from build123d import *

# Parameters (mm, degrees)
SKETCH_1_R      = 11.5
SKETCH_1_R_2    = 1.6
SKETCH_1_R_3    = 4.3
SKETCH_1_R_4    = 2.5
EXTRUDE_3_DEPTH = 4
SKETCH_4_W      = 42
SKETCH_4_H      = 2.6
EXTRUDE_4_DEPTH = 6
SKETCH_4_3_W    = 42
SKETCH_4_3_H    = 2.6
EXTRUDE_5_DEPTH = 5
CHAMFER_3_SIZE  = 4
CHAMFER_3_SIZE2 = 22
CHAMFER_4_SIZE  = 22
CHAMFER_4_SIZE2 = 4


with BuildPart() as part:
    # Sketch 1 → Extrude 3 (new body)
    with BuildSketch(Plane.XY):
        with BuildLine():
            Line((-21, 24), (35, 24))
            ThreePointArc((35, 24), (39.242640687, 22.242640687), (41, 18))
            Line((41, 18), (41, -18))
            ThreePointArc((41, -18), (39.242640687, -22.242640687), (35, -24))
            Line((35, -24), (-21, -24))
            Line((-21, -24), (-21, -9.797958971))
            ThreePointArc((-21, -9.797958971), (-21.445079401, -7.530172133), (-22.714285714, -5.598833698))
            ThreePointArc((-22.714285714, -5.598833698), (-25, 0), (-22.714285714, 5.598833698))
            ThreePointArc((-22.714285714, 5.598833698), (-21.445079401, 7.530172133), (-21, 9.797958971))
            Line((-21, 9.797958971), (-21, 24))
        make_face()
        Circle(SKETCH_1_R, mode=Mode.SUBTRACT)
        with Locations((15.5, 15.5)):
            Circle(SKETCH_1_R_2, mode=Mode.SUBTRACT)
        with Locations((15.5, -15.5)):
            Circle(SKETCH_1_R_2, mode=Mode.SUBTRACT)
        with Locations((-15.5, -15.5)):
            Circle(SKETCH_1_R_2, mode=Mode.SUBTRACT)
        with Locations((-15.5, 15.5)):
            Circle(SKETCH_1_R_2, mode=Mode.SUBTRACT)
        with Locations((-17, 0)):
            Circle(SKETCH_1_R_3, mode=Mode.SUBTRACT)
        with Locations((31, 15.5)):
            Circle(SKETCH_1_R_4, mode=Mode.SUBTRACT)
        with Locations(Location((31, -15.5, 0), (0, 0, 180))):
            Circle(SKETCH_1_R_4, mode=Mode.SUBTRACT)
    extrude(amount=EXTRUDE_3_DEPTH)

    # Sketch 4 → Extrude 4 (add)
    with BuildSketch(Plane.XY.offset(4)):
        with Locations((0, 22.7)):
            Rectangle(SKETCH_4_W, SKETCH_4_H)
        with Locations((0, -22.7)):
            Rectangle(SKETCH_4_W, SKETCH_4_H)
    extrude(amount=EXTRUDE_4_DEPTH)

    # Sketch 4_3 → Extrude 5 (add)
    with BuildSketch(Plane.XY.offset(4)):
        with Locations((0, 22.7)):
            Rectangle(SKETCH_4_3_W, SKETCH_4_3_H)
        with BuildLine():
            Line((29, 8), (33, 8))
            ThreePointArc((33, 8), (33.707106781, 7.707106781), (34, 7))
            Line((34, 7), (34, -7))
            ThreePointArc((34, -7), (33.707106781, -7.707106781), (33, -8))
            Line((33, -8), (29, -8))
            ThreePointArc((29, -8), (28.292893219, -7.707106781), (28, -7))
            Line((28, -7), (28, 7))
            ThreePointArc((28, 7), (28.292893219, 7.707106781), (29, 8))
        make_face()
        with Locations((0, -22.7)):
            Rectangle(SKETCH_4_3_W, SKETCH_4_3_H)
    extrude(amount=EXTRUDE_5_DEPTH)

    # Chamfer 3
    chamfer_3_edges = [part.edges().sort_by_distance(p)[0] for p in [
        (-21, 22.7, 10),
    ]]
    chamfer_3_side = [part.faces().sort_by_distance(p)[0] for p in [
        (-21, 18.1487822, 3.077226594),
    ]]
    chamfer(chamfer_3_edges, length=CHAMFER_3_SIZE, length2=CHAMFER_3_SIZE2, reference=chamfer_3_side[0])

    # Chamfer 4
    chamfer_4_edges = [part.edges().sort_by_distance(p)[0] for p in [
        (-21, -22.7, 10),
    ]]
    chamfer_4_side = [part.faces().sort_by_distance(p)[0] for p in [
        (0, -22.7, 10),
    ]]
    chamfer(chamfer_4_edges, length=CHAMFER_4_SIZE, length2=CHAMFER_4_SIZE2, reference=chamfer_4_side[0])


solid = part.part
Design review of the part built by this model. Coordinates are the model's own, in mm. A direction names the side the tool comes from. Give positions to 0.01 mm unless a question says otherwise; leave off trailing zeros. Loops run counter-clockwise (first coordinate to the right, second up) from the corner with the lowest first, then second, coordinate; pieces in that order, holes last. Notation, with made-up numbers: (0, 41) -> (43, 41) arc R21 ccw to (43, 62) -> close; hole circle Ø10 at (-1.75, -29). An arc over 180 degrees is marked (long way). One line per question, with ' | ' between items. Start each with the question number.
(1) For line 1 (Y direction, x = 15.5, z = 1.7); line 2 (Y direction, x = 31, z = 1.1); line 3 (Y direction, x = 4.5, z = 5.5), list the stretches that pass through material, from the lowest coordinate up.
(2) Draft analysis for pull direction X (two halves, no side actions). For faces 1 (the face through (-21, 17, 2)), 2 (the face through (-16.68, -14.42, 1.97)), 3 (the face through (16, 0, 4)), state which applies: +X half, -X half, draft (parallel to the pull), parting line (faces both ways), or undercut.
(3) We need section A-A (x = 31). State the section outline as (y, z) points.
(4) We need section D-D (y = 15.5). State the section outline as (x, z) points, and give its area (3 significant figures).
(5) We need section B-B (z = 2). State how many separate pieces and enclosed holes the cut face has, and give its area (3 significant figures).
(6) Insertion check: P1, Ø2, axis at y = 5, z = 3, coming from the -X side; P2, Ø1, axis at x = 14.5, y = -5.5, coming from the +Z side; P3, Ø0.8, axis at y = -23, z = 7, coming from the +X side. Each pin has a flat end and moves straight along its axis. Give the tip position at first contact, or say it passes through.
(7) We need section C-C (y = 0). State the section outline as (x, z) points.
(8) For faces 4 (the face through (4, 21.4, 6)), 5 (the face through (33.5, -15.6, 2)), 6 (the face through (16, 0, 0)), 7 (the face through (31, -8, 6)), 8 (the face through (34, 0, 6)), list the 3-axis set-ups (+Z, -Z, +X, -X, +Y, -Y) from which the entire face can be reached by the end or side of a thin tool; tool diameter is ignored.
The answers:
1) line 1: y = -24 to -17.1, -13.9 to 13.9, 17.1 to 24 | line 2: y = -24 to -18, -13 to 13, 18 to 24 | line 3: y = -24 to -21.4, 21.4 to 24
2) face 1: -X half | face 2: undercut | face 3: draft
3) outline: (-24, 0) -> (-18, 0) -> (-18, 4) -> (-24, 4) -> close; (-13, 0) -> (13, 0) -> (13, 4) -> (8, 4) -> (8, 9) -> (-8, 9) -> (-8, 4) -> (-13, 4) -> close; (18, 0) -> (24, 0) -> (24, 4) -> (18, 4) -> close
4) outline: (-21, 0) -> (-17.1, 0) -> (-17.1, 4) -> (-21, 4) -> close; (-13.9, 0) -> (13.9, 0) -> (13.9, 4) -> (-13.9, 4) -> close; (17.1, 0) -> (28.5, 0) -> (28.5, 4) -> (17.1, 4) -> close; (33.5, 0) -> (41, 0) -> (41, 4) -> (33.5, 4) -> close | area: 202 mm^2
5) separate pieces: 1 | enclosed holes: 8 | area: 2,460 mm^2
6) P1: stops at x = -23.93 | P2: stops at z = 4 | P3: stops at x = 21
7) outline: (-25, 0) -> (-21.3, 0) -> (-21.3, 4) -> (-25, 4) -> close; (-12.7, 0) -> (-11.5, 0) -> (-11.5, 4) -> (-12.7, 4) -> close; (11.5, 0) -> (41, 0) -> (41, 4) -> (34, 4) -> (34, 9) -> (28, 9) -> (28, 4) -> (11.5, 4) -> close
8) face 4: +Z, +X, -X | face 5: +Z, -Z | face 6: -Z, +X, -X, +Y, -Y | face 7: +Z, +X, -X, -Y | face 8: +Z, +X, +Y, -Y
